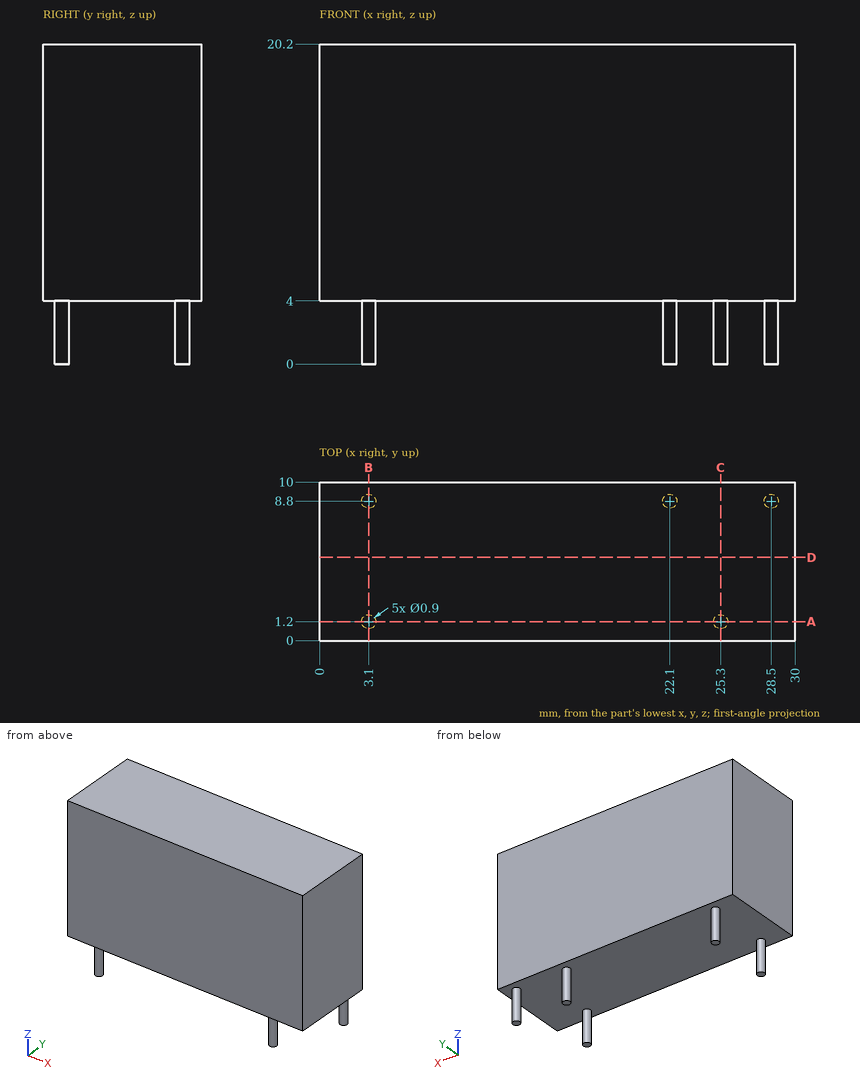
The drawing under review shows one solid part. Ordinate dimensions are in mm from its lowest x, y, z. Round coordinates to 2 decimals unless told otherwise and drop trailing zeros. Write each loop counter-clockwise with the first axis right and the second up, starting at its lowest first coordinate (ties: lowest second). Pieces come first, ordered by that corner, then holes. Notation, with made-up numbers: (30.25, -3.75) - (78.25, -3.75) arc R18 ccw to (78.25, 11.25) - close; hole circle Ø7 at (54.5, -18). An arc over 180 degrees is marked (long way). Use a Markdown table: item, result. Add a question column.
1. Clearance check with a flat-ended pin moving along its axis: pin 1 (1 mm diameter, centred on x = 9, y = 6, fed in from -Z). State where the tip first meets the part, or that it passes through.
2. We need section D-D (y = 5.25). State the section outline as (x, z) points, then the cut area to 3 significant figures.
3. We need section B-B (x = 3.1). State the section outline as (y, z) points, then the cut area to 3 significant figures.
4. We need section A-A (y = 1.2). State the section outline as (x, z) points.
5. We need section C-C (x = 25.3). State the section outline as (y, z) points, then the cut area to 3 significant figures.
6. Wall thickness on probe 1 along Z at (x, y) = (4.5, 6); probe 2 along Y at (x, z) = (22.25, 3.25): over which ranges is each line inside the solid? List them lowest first.
Output:
| question | item | result |
|---|---|---|
| 1 | pin 1 | stops at z = 4 |
| 2 | outline | (0, 4) - (30, 4) - (30, 20.2) - (0, 20.2) - close |
| 2 | area | 486 mm2 |
| 3 | outline | (0, 4) - (0.75, 4) - (0.75, 0) - (1.65, 0) - (1.65, 4) - (8.35, 4) - (8.35, 0) - (9.25, 0) - (9.25, 4) - (10, 4) - (10, 20.2) - (0, 20.2) - close |
| 3 | area | 169 mm2 |
| 4 | outline | (0, 4) - (2.65, 4) - (2.65, 0) - (3.55, 0) - (3.55, 4) - (24.85, 4) - (24.85, 0) - (25.75, 0) - (25.75, 4) - (30, 4) - (30, 20.2) - (0, 20.2) - close |
| 5 | outline | (0, 4) - (0.75, 4) - (0.75, 0) - (1.65, 0) - (1.65, 4) - (10, 4) - (10, 20.2) - (0, 20.2) - close |
| 5 | area | 166 mm2 |
| 6 | probe 1 | z = 4 to 20.2 |
| 6 | probe 2 | y = 8.38 to 9.22 |
